The model under review builds one solid part; all positions refer to its coordinate system, in mm. Face numbers are marked on the shaded views. A direction names the side the tool comes from. Give positions to 0.01 mm unless a question says otherwise; leave off trailing zeros. Order: outer loops, then holes, each group sorted by start corner. A loop starts at its lowest first (then second) coordinate and runs counter-clockwise, first axis right, second up. Notation, with made-up numbers: (-21.5, -29.75) - (0.5, -29.75) arc R22 ccw to (0.5, -16.75) - close; hole circle Ø10 at (29, 63.25). An arc over 180 degrees is marked (long way). Write item = value, one per line. Start each with the question number.
1. We need section A-A, the plane y = 38. State how many separate pieces and enclosed holes the cut face has, and give its area (3 significant figures).
2. We need section C-C, the plane x = 44. Give the boundary of the cut face in (y, z) (3 decimals).
3. Machinability: for the marked faces 1, 2, 3, 4 and 5, which of the approach directions +Z, -Z, +X, -X, +Y, -Y give a long, thin tool a straight path to every point of the face, cutting with its end or side? Answer none if there is none.
4. Wall thickness on probe 1 along Y at (x, z) = (45, 5); probe 2 along X at (y, z) = (61, 1); probe 3 along Z at (x, y) = (57, 41) (3 decimals): over which ranges is each line inside the solid? List them lowest first.
5. For P1, Ø1, axis at y = 60, z = 1, coming from the +X side; P2, Ø3.5, axis at x = 1, z = 1, coming from the +Y side; P3, Ø4, axis at y = 14.5, z = 9.5, coming from the -X side (3 decimals); P4, Ø4, axis at x = 40, y = 20, coming from the -Z side (3 decimals), all flat-tipped, find the tip position at first contact; note any pin that passes through.
6. We need section D-D, the plane x = 13. Give the boundary of the cut face in (y, z) (3 decimals).
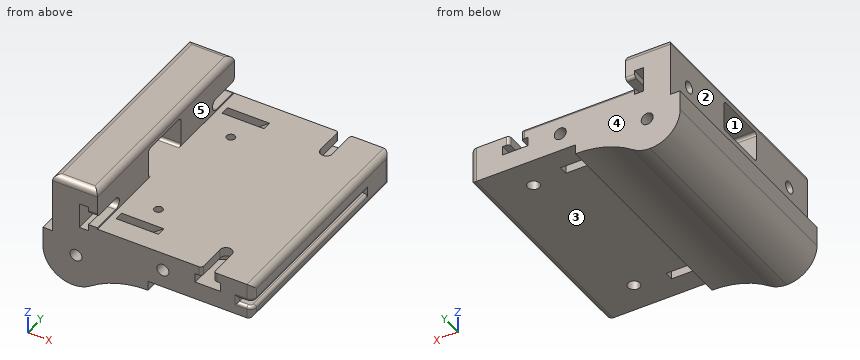
from build123d import *

# Parameters (mm, degrees)
BOSS_EXTRUDE1_DEPTH = 75
SKETCH2_R           = 2
CUT_EXTRUDE1_DEPTH  = 15
SKETCH4_R           = 2
CUT_EXTRUDE2_DEPTH  = 12
SKETCH3_R           = 2
CUT_EXTRUDE3_DEPTH  = 75
CUT_EXTRUDE4_START  = -3
CUT_EXTRUDE4_DEPTH  = 3
CUT_EXTRUDE5_START  = -3
CUT_EXTRUDE5_DEPTH  = 3
CUT_EXTRUDE6_START  = -3
CUT_EXTRUDE6_DEPTH  = 3
CUT_EXTRUDE7_START  = -3
CUT_EXTRUDE7_DEPTH  = 3
CUT_EXTRUDE12_START = -7
CUT_EXTRUDE12_DEPTH = 3
CUT_EXTRUDE14_START = -7
CUT_EXTRUDE14_DEPTH = 3
FILLET2_START       = 9
FILLET2_DEPTH       = 4.666666667
FILLET2_START_2     = 4
FILLET2_2_DEPTH     = 39
FILLET3_R           = 2
SKETCH10_W          = 1.75
SKETCH10_H          = 62.75
CUT_EXTRUDE9_DEPTH  = 5
FILLET4_R           = 1
SKETCH11_W          = 10.2
SKETCH11_H          = 17.7
CUT_EXTRUDE10_DEPTH = 15
SKETCH12_R          = 1.397
CUT_EXTRUDE11_DEPTH = 10
FILLET5_R           = 1


with BuildPart() as part:
    # Sketch1 → Boss-Extrude1 (new body)
    with BuildSketch(Plane(origin=(0, 0, 0), x_dir=(1, 0, 0), z_dir=(0, 1, 0))):
        with BuildLine():
            Line((-6.825, -6.666666667), (-6.825, -26.666666667))
            Line((-6.825, -26.666666667), (8.175, -26.666666667))
            Line((8.175, -26.666666667), (8.175, -13.175))
            Line((8.175, -13.175), (60, -13.175))
            Line((60, -13.175), (60, -1.175))
            Line((60, -1.175), (25, -1.175))
            Line((25, -1.175), (25, 2))
            ThreePointArc((25, 2), (14.923352523, 3.572976633), (5.805515239, 8.142235123))
            ThreePointArc((5.805515239, 8.142235123), (3.047757271, 9.524241472), (0, 10))
            ThreePointArc((0, 10), (-7.071067812, 7.071067812), (-10, 0))
            Line((-10, 0), (-10, -6.666666667))
            Line((-10, -6.666666667), (-6.825, -6.666666667))
        make_face()
    extrude(amount=BOSS_EXTRUDE1_DEPTH)

    # Sketch2 → Cut-Extrude1 (cut)
    with BuildSketch(Plane.ZY.offset(6.825)):
        with Locations((15.666666667, 65)):
            Circle(SKETCH2_R)
    cut_extrude1 = extrude(amount=-CUT_EXTRUDE1_DEPTH, mode=Mode.SUBTRACT)

    # Sketch4 → Cut-Extrude2 (cut)
    with BuildSketch(Plane(origin=(0, 0, 1.175), x_dir=(-1, 0, 0), z_dir=(0, 0, -1))):
        with Locations((-45, 65)):
            Circle(SKETCH4_R)
    cut_extrude2 = extrude(amount=-CUT_EXTRUDE2_DEPTH, mode=Mode.SUBTRACT)

    # Sketch3 → Cut-Extrude3 (cut)
    with BuildSketch(Plane(origin=(0, 75, 0), x_dir=(1, 0, 0), z_dir=(0, 1, 0))):
        with Locations(Location((1, -1, 0), (0, 0, 270))):
            Circle(SKETCH3_R)
        with Locations(Location((30, -7.175, 0), (0, 0, 270))):
            Circle(SKETCH3_R)
    extrude(amount=-CUT_EXTRUDE3_DEPTH, mode=Mode.SUBTRACT)

    # Sketch5 → Cut-Extrude4 (cut)
    with BuildSketch(Plane(origin=(8.175, 0, 0), x_dir=(0, 0, -1), z_dir=(1, 0, 0)).offset(CUT_EXTRUDE4_START)):
        Polygon((-19.885416667, 62.564303552), (-15.666666667, 60.128607104), (-11.447916667, 62.564303552), (-11.447916667, 75), (-19.885416667, 75), align=None)
    cut_extrude4 = extrude(amount=-CUT_EXTRUDE4_DEPTH, mode=Mode.SUBTRACT)

    # Sketch6 → Cut-Extrude5 (cut)
    with BuildSketch(Plane(origin=(8.175, 0, 0), x_dir=(0, 0, -1), z_dir=(1, 0, 0)).offset(CUT_EXTRUDE5_START)):
        with BuildLine():
            Line((-13.666666667, 65), (-13.666666667, 75))
            Line((-13.666666667, 75), (-17.666666667, 75))
            Line((-17.666666667, 75), (-17.666666667, 65))
            ThreePointArc((-17.666666667, 65), (-15.666666667, 67), (-13.666666667, 65))
        make_face()
    cut_extrude5 = extrude(amount=CUT_EXTRUDE5_DEPTH, mode=Mode.SUBTRACT)

    # Sketch7 → Cut-Extrude6 (cut)
    with BuildSketch(Plane.XY.offset(13.175).offset(CUT_EXTRUDE6_START)):
        Polygon((40.78125, 62.564303552), (45, 60.128607104), (49.21875, 62.564303552), (49.21875, 75), (40.78125, 75), align=None)
    cut_extrude6 = extrude(amount=-CUT_EXTRUDE6_DEPTH, mode=Mode.SUBTRACT)

    # Sketch8 → Cut-Extrude7 (cut)
    with BuildSketch(Plane.XY.offset(13.175).offset(CUT_EXTRUDE7_START)):
        with BuildLine():
            Line((47, 65), (47, 75))
            Line((47, 75), (43, 75))
            Line((43, 75), (43, 65))
            ThreePointArc((43, 65), (45, 67), (47, 65))
        make_face()
    cut_extrude7 = extrude(amount=CUT_EXTRUDE7_DEPTH, mode=Mode.SUBTRACT)

    # Sketch13 → Cut-Extrude12 (cut)
    with BuildSketch(Plane.XZ.offset(CUT_EXTRUDE12_START)):
        Polygon((-2.893869279, -1.927157459), (1.588058081, -3.835768444), (5.48192736, -0.908610985), (24.216737808, 13.175), (10.175, 13.175), (0.411941919, 5.835768444), (-3.48192736, 2.908610985), align=None)
    cut_extrude12 = extrude(amount=-CUT_EXTRUDE12_DEPTH, mode=Mode.SUBTRACT)

    # Sketch16 → Cut-Extrude14 (cut)
    with BuildSketch(Plane(origin=(0, 75, 0), x_dir=(1, 0, 0), z_dir=(0, 1, 0)).offset(CUT_EXTRUDE14_START)):
        Polygon((25.78125, -4.739303552), (25.78125, -1.175), (34.21875, -1.175), (34.21875, -4.739303552), (34.21875, -9.610696448), (30, -12.046392896), (25.78125, -9.610696448), align=None)
    cut_extrude14 = extrude(amount=-CUT_EXTRUDE14_DEPTH, mode=Mode.SUBTRACT)

    # Mirror2: Cut-Extrude1, Cut-Extrude2, Cut-Extrude4, Cut-Extrude5, Cut-Extrude6, Cut-Extrude7, Cut-Extrude12, Cut-Extrude14 across plane
    add(cut_extrude1.mirror(Plane.ZX.offset(37.5)), mode=Mode.SUBTRACT)
    add(cut_extrude2.mirror(Plane.ZX.offset(37.5)), mode=Mode.SUBTRACT)
    add(cut_extrude4.mirror(Plane.ZX.offset(37.5)), mode=Mode.SUBTRACT)
    add(cut_extrude5.mirror(Plane.ZX.offset(37.5)), mode=Mode.SUBTRACT)
    add(cut_extrude6.mirror(Plane.ZX.offset(37.5)), mode=Mode.SUBTRACT)
    add(cut_extrude7.mirror(Plane.ZX.offset(37.5)), mode=Mode.SUBTRACT)
    add(cut_extrude12.mirror(Plane.ZX.offset(37.5)), mode=Mode.SUBTRACT)
    add(cut_extrude14.mirror(Plane.ZX.offset(37.5)), mode=Mode.SUBTRACT)

    # Fillet2: read off the stored shape, not the designer's step
    # Fillet2 outline → Fillet2 (cut)
    with BuildSketch(Plane.XY.offset(FILLET2_START)):
        with BuildLine():
            Line((47, 1), (47, 0))
            Line((47, 0), (48, 0))
            ThreePointArc((48, 0), (47.292893219, 0.292893219), (47, 1))
        make_face()
        with BuildLine():
            Line((48, 75), (47, 75))
            Line((47, 75), (47, 74))
            ThreePointArc((47, 74), (47.292893219, 74.707106781), (48, 75))
        make_face()
        with BuildLine():
            Line((43, 75), (42, 75))
            ThreePointArc((42, 75), (42.707106781, 74.707106781), (43, 74))
            Line((43, 74), (43, 75))
        make_face()
        with BuildLine():
            ThreePointArc((43, 1), (42.707106781, 0.292893219), (42, 0))
            Line((42, 0), (43, 0))
            Line((43, 0), (43, 1))
        make_face()
    extrude(amount=FILLET2_DEPTH, mode=Mode.SUBTRACT)

    # Fillet2 2 outline → Fillet2 2 (cut)
    with BuildSketch(Plane.YZ.offset(FILLET2_START_2)):
        with BuildLine():
            Line((74, 17.666666667), (75, 17.666666667))
            Line((75, 17.666666667), (75, 18.666666667))
            ThreePointArc((75, 18.666666667), (74.707106782, 17.959559886), (74, 17.666666667))
        make_face()
        with BuildLine():
            ThreePointArc((74, 13.666666667), (74.707106781, 13.373773448), (75, 12.666666667))
            Line((75, 12.666666667), (75, 13.666666667))
            Line((75, 13.666666667), (74, 13.666666667))
        make_face()
        with BuildLine():
            ThreePointArc((1, 17.666666667), (0.292893218, 17.959559886), (0, 18.666666667))
            Line((0, 18.666666667), (0, 17.666666667))
            Line((0, 17.666666667), (1, 17.666666667))
        make_face()
    extrude(amount=FILLET2_2_DEPTH, mode=Mode.SUBTRACT)

    # Fillet3
    fillet3_edges = [part.edges().sort_by_distance(p)[0] for p in [
        (60, 0, 7.175),
        (0.675, 0, 26.666666667),
        (60, 37.5, 1.175),
        (60, 37.5, 13.175),
        (8.175, 37.5, 26.666666667),
        (-6.825, 37.5, 26.666666667),
        (0.675, 75, 26.666666667),
        (60, 75, 7.175),
    ]]
    fillet(fillet3_edges, radius=FILLET3_R)

    # Sketch10 → Cut-Extrude9 (cut)
    with BuildSketch(Plane(origin=(60, 0, 0), x_dir=(0, 0, -1), z_dir=(1, 0, 0))):
        with Locations((-6.175, 31.375)):
            Rectangle(SKETCH10_W, SKETCH10_H)
    extrude(amount=-CUT_EXTRUDE9_DEPTH, mode=Mode.SUBTRACT)

    # Fillet4
    fillet4_edges = [part.edges().sort_by_distance(p)[0] for p in [
        (59.414213562, 0.585786438, 7.05),
        (59.414213562, 0.585786438, 5.3),
        (60, 32.375, 7.05),
        (60, 32.375, 5.3),
        (55, 0, 6.175),
        (56.5, 0, 5.3),
        (56.5, 0, 7.05),
    ]]
    fillet(fillet4_edges, radius=FILLET4_R)

    # Sketch11 → Cut-Extrude10 (cut)
    with BuildSketch(Plane(origin=(8.175, 0, 0), x_dir=(0, 0, -1), z_dir=(1, 0, 0))):
        with Locations((-18.275, 36.85)):
            Rectangle(SKETCH11_W, SKETCH11_H)
    extrude(amount=-CUT_EXTRUDE10_DEPTH, mode=Mode.SUBTRACT)

    # Sketch12 → Cut-Extrude11 (cut)
    with BuildSketch(Plane.XY.offset(13.175)):
        with Locations((18.175, 17)):
            Circle(SKETCH12_R)
        with Locations((18.175, 56.7)):
            Circle(SKETCH12_R)
    extrude(amount=-CUT_EXTRUDE11_DEPTH, mode=Mode.SUBTRACT)

    # Fillet5
    fillet5_edges = [part.edges().sort_by_distance(p)[0] for p in [
        (0.675, 45.7, 13.175),
        (0.675, 28, 13.175),
        (0.675, 28, 23.375),
        (0.675, 45.7, 23.375),
    ]]
    fillet(fillet5_edges, radius=FILLET5_R)


solid = part.part
Model answer:
q1.separate_pieces = 2
q1.enclosed_holes = 2
q1.area = 1,080 mm2
q2.outline = (0, 1.175) - (8.268, 1.175) - (8.268, 7.175) - (0, 7.175) - close; (11.732, 1.175) - (63.268, 1.175) - (63.268, 7.175) - (60.706, 7.175) - (60.706, 10.175) - (63.268, 10.175) - (63.268, 13.175) - (11.732, 13.175) - (11.732, 10.175) - (14.294, 10.175) - (14.294, 7.175) - (11.732, 7.175) - close; (66.732, 1.175) - (75, 1.175) - (75, 7.175) - (66.732, 7.175) - close
q3.face_1 = +X, -X
q3.face_2 = +Z, -X, +Y, -Y
q3.face_3 = -Z, +X, +Y, -Y
q3.face_4 = +Z, -Z, +X, -X, +Y
q3.face_5 = +Z, +X, +Y, -Y
q4.probe_1 = 0 to 8, 12 to 63, 67 to 75
q4.probe_2 = -10 to -1, 3 to 25
q4.probe_3 = 1.175 to 5.3, 7.05 to 13.175
q5.P1 = 59.09
q5.P2 = through
q5.P3 = -6.825
q5.P4 = 1.175
q6.outline = (0, -4.255) - (75, -4.255) - (75, 12.667) arc R1 ccw to (74.861, 13.175) - (68, 13.175) - (68, 4.743) - (65, 4.743) - (65, 13.175) - (10, 13.175) - (10, 4.743) - (7, 4.743) - (7, 13.175) - (0, 13.175) - close
